Work out the finished part from the listing and answer in its coordinate system (mm). A direction names the side the tool comes from. Give positions to 0.01 mm unless a question says otherwise; leave off trailing zeros. Loops run counter-clockwise (first coordinate to the right, second up) from the corner with the lowest first, then second, coordinate; pieces in that order, holes last. Notation, with made-up numbers: (-6, 81) - (30, 81) arc R16 ccw to (30, 93) - close; hole circle Ø1 at (27, 56). An arc over 180 degrees is marked (long way). Use CSV: the item, a comma, the result in double quotes.
from build123d import *

# Parameters (mm, degrees)
F0_W     = 65
F0_H     = 40
F1_DEPTH = 4
F2_R     = 5
F3_DEPTH = 25
F4_R     = 1.25
F5_DEPTH = 5
F6_R     = 2
F7_R     = 2.5
F8_DEPTH = 25


with BuildPart() as f1:
    # F0 (on Top) → F1 (new body)
    with BuildSketch(Plane.XY):
        with Locations((32.639029, 20.218261)):
            Rectangle(F0_W, F0_H)
    extrude(amount=F1_DEPTH)

    # F2 (on face) → F3 (cut)
    with BuildSketch(Plane.XY.offset(4)):
        with Locations((32.639029, 20.218261)):
            Circle(F2_R)
    extrude(amount=-F3_DEPTH, mode=Mode.SUBTRACT)

    # F4 (on face) → F5 (join)
    with BuildSketch(Plane.XY.offset(4)):
        with BuildLine():
            ThreePointArc((51.389029, 32.218261), (50.139029, 33.468261), (48.889029, 32.218261))
            ThreePointArc((48.889029, 32.218261), (50.139029, 30.968261), (51.389029, 32.218261))
        make_face()
        with Locations((15.139029, 32.218261)):
            Circle(F4_R)
    extrude(amount=F5_DEPTH)

    # F6
    f6_edges = [f1.edges().sort_by_distance(p)[0] for p in [
        (0.139029, 0.218261, 2),
        (65.139029, 0.218261, 2),
        (65.139029, 40.218261, 2),
        (0.139029, 40.218261, 2),
    ]]
    fillet(f6_edges, radius=F6_R)

    # F7 (on face) → F8 (cut)
    with BuildSketch(Plane.XY.offset(4)):
        with Locations((3.639029, 36.718261)):
            Circle(F7_R)
        with Locations((3.639029, 3.718261)):
            Circle(F7_R)
        with BuildLine():
            ThreePointArc((64.139029, 3.718261), (61.639029, 6.218261), (59.139029, 3.718261))
            ThreePointArc((59.139029, 3.718261), (61.639029, 1.218261), (64.139029, 3.718261))
        make_face()
        with BuildLine():
            ThreePointArc((64.139029, 36.718261), (61.639029, 39.218261), (59.139029, 36.718261))
            ThreePointArc((59.139029, 36.718261), (61.639029, 34.218261), (64.139029, 36.718261))
        make_face()
    extrude(amount=-F8_DEPTH, mode=Mode.SUBTRACT)


solid = f1.part
Item 1: Given P1, Ø8, axis at x = 3.64, y = 36.72, coming from the +Z side; P2, Ø1.5, axis at x = 43, z = 5, coming from the -Y side, each flat-ended and moving along its own axis, determine where each tip first touches the part or whether it passes through.
Determined:
P1,"stops at z = 4"
P2,"passes through"
Item 2: Find the intervals of material crossed by line 1 (X direction, y = 4, z = 1.25); line 2 (Y direction, x = 60, z = 3.25); line 3 (Z direction, x = 56, y = 4.5), in increasing order.
Determined:
line 1,"x = 0.14 to 1.15, 6.12 to 59.15, 64.12 to 65.14"
line 2,"y = 0.22 to 1.83, 5.61 to 34.83, 38.61 to 40.22"
line 3,"z = 0 to 4"
Item 3: A cutting plane is placed at D-D on z = 2.5. Determine the outline of the cut face in (x, y).
Determined:
outline,"(0.14, 2.22) arc R2 ccw to (2.14, 0.22) - (63.14, 0.22) arc R2 ccw to (65.14, 2.22) - (65.14, 38.22) arc R2 ccw to (63.14, 40.22) - (2.14, 40.22) arc R2 ccw to (0.14, 38.22) - close; hole circle Ø5 at (3.64, 3.72); hole circle Ø5 at (3.64, 36.72); hole circle Ø10 at (32.64, 20.22); hole circle Ø5 at (61.64, 3.72); hole circle Ø5 at (61.64, 36.72)"
Item 4: A cutting plane is placed at C-C on z = 7. Determine the outline of the cut face in (x, y).
Determined:
outline,"circle Ø2.5 at (15.14, 32.22); circle Ø2.5 at (50.14, 32.22)"
Item 5: A cutting plane is placed at B-B on y = 24.5. Determine the outline of the cut face in (x, z).
Determined:
outline,"(0.14, 0) - (30.06, 0) - (30.06, 4) - (0.14, 4) - close; (35.22, 0) - (65.14, 0) - (65.14, 4) - (35.22, 4) - close"
Item 6: The mould has two halves that part along X. Classify faces 3 (the cylindrical face through (59.254, 35.967, 2.028)), 4 (the flat face through (25, 20, 0)), 5 (the cylindrical face through (64.538, 39.648, 2.028)): pulls with the +X half, pulls with the -X half, needs draft (parallel to the pull), parting line crosses it, or undercut.
Determined:
face 3,"undercut"
face 4,"needs draft"
face 5,"pulls with the +X half"
Item 7: For faces 1 (the flat face through (32, 0.218, 2)), 2 (the cylindrical face through (48.947, 31.843, 6.465)), determine the directions among +Z, -Z, +X, -X, +Y, -Y from which every point of the face is accessible in a straight line to the end or side of a thin tool.
Determined:
face 1,"+Z, -Z, +X, -X, -Y"
face 2,"+Z"
Item 8: A cutting plane is placed at A-A on x = 32. Determine the outline of the cut face in (y, z).
Determined:
outline,"(0.22, 0) - (15.26, 0) - (15.26, 4) - (0.22, 4) - close; (25.18, 0) - (40.22, 0) - (40.22, 4) - (25.18, 4) - close"
